```python
from build123d import *

# Parameters (mm, degrees)
F0_W      = 2032
F0_H      = 812.8
F1_DEPTH  = 914.4
F4_DEPTH  = 1955.8
F3_W      = 1879.6
F3_H      = 330.2
F5_DEPTH  = 736.6
F6_W      = 660.4
F6_H      = 241.3
F7_DEPTH  = 736.6
F8_W      = 76.2
F8_H      = 660.4
F10_R     = 76.2
F11_DEPTH = 76.2
F12_DEPTH = 50.8


with BuildPart() as f1:
    # F0 (on Top) → F1 (new body)
    with BuildSketch(Plane.XY):
        Rectangle(F0_W, F0_H)
    extrude(amount=F1_DEPTH)

    # F2 (on face) → F4 (cut)
    with BuildSketch(Plane.YZ.offset(1016)):
        with BuildLine():
            Line((330.2, 63.5), (330.2, 304.8))
            ThreePointArc((330.2, 304.8), (0, 381), (-330.2, 304.8))
            Line((-330.2, 304.8), (-330.2, 63.5))
            Line((-330.2, 63.5), (330.2, 63.5))
        make_face()
    extrude(amount=-F4_DEPTH, mode=Mode.SUBTRACT)

    # F3 (on face) → F5 (cut)
    with BuildSketch(Plane.XZ.offset(406.4)):
        with Locations((0, 698.5)):
            Rectangle(F3_W, F3_H)
    extrude(amount=-F5_DEPTH, mode=Mode.SUBTRACT)

    # F6 (on face) → F7 (cut)
    with BuildSketch(Plane.XZ.offset(406.4)):
        with Locations((-609.6, 184.15)):
            Rectangle(F6_W, F6_H)
        with BuildLine():
            ThreePointArc((-279.4, 304.8), (-609.6, 381), (-939.8, 304.8))
            Line((-939.8, 304.8), (-279.4, 304.8))
        make_face()
    extrude(amount=-F7_DEPTH, mode=Mode.SUBTRACT)

    # F8 (on face) → F9 (join, up to the next surface of F1)
    with BuildSketch(Plane.XY.offset(63.5)):
        with Locations((977.9, 0)):
            Rectangle(F8_W, F8_H)
    extrude(until=Until.NEXT)

    # F10 (on face) → F11 (cut, through all)
    with BuildSketch(Plane.YZ.offset(1016)):
        with Locations((0, 152.4)):
            Circle(F10_R)
    extrude(amount=-F11_DEPTH, mode=Mode.SUBTRACT)

    # F12 (cut): a face of the model
    f12_faces = [f1.faces().sort_by_distance(p)[0] for p in [
        (0, 0, 914.4),
    ]]
    extrude(f12_faces, amount=-F12_DEPTH, mode=Mode.SUBTRACT)


solid = f1.part
```
For this review, take the finished solid that the model builds, in its own axes (mm). A direction names the side the tool comes from. Give positions to 0.01 mm unless a question says otherwise; leave off trailing zeros. Write each loop counter-clockwise with the first axis right and the second up, starting at its lowest first coordinate (ties: lowest second). Pieces come first, ordered by that corner, then holes. Notation, with made-up numbers: M 89.5,43 L 147.5,43 A30 ccw 147.5,76 Z; hole C 26.25,-11.5 d5. An arc over 180 degrees is marked long. Answer as CSV lines item,"result".
1. Consider section C-C, the plane y = -196. Write out the cut boundary in (x, z), then the cut area to 3 significant figures.
Findings:
outline,"M -1016,0 L 1016,0 L 1016,863.6 L 939.8,863.6 L 939.8,533.4 L -939.8,533.4 L -939.8,863.6 L -1016,863.6 Z; hole M -939.8,63.5 L 939.8,63.5 L 939.8,355.06 L -413.6,355.06 A753.53 ccw -805.6,355.06 L -939.8,355.06 Z"
area,"579,000 mm2"
2. Wall thickness on line 1 (X direction, y = -156.5, z = 250); line 2 (Z direction, x = -587, y = 197); line 3 (Y direction, x = -53.5, z = 178.5): over which ranges is each line inside the solid? List them lowest first.
Findings:
line 1,"x = -1016 to -939.8, 939.8 to 1016"
line 2,"z = 0 to 63.5, 380.66 to 533.4"
line 3,"y = -406.4 to -330.2, 330.2 to 406.4"
3. Consider section D-D, the plane z = 683. Write out the cut boundary in (x, y).
Findings:
outline,"M -1016,-406.4 L -939.8,-406.4 L -939.8,330.2 L 939.8,330.2 L 939.8,-406.4 L 1016,-406.4 L 1016,406.4 L -1016,406.4 Z"
4. For faces 4 (the flat face through (-939.8, -43, 220)), 5 (the flat face through (-279.4, -369, 182)), 6 (the flat face through (-13, -43, 533.4)), list the 3-axis set-ups (+Z, -Z, +X, -X, +Y, -Y) from which the entire face can be reached by the end or side of a thin tool; tool diameter is ignored.
Findings:
face 4,"none"
face 5,"-Y"
face 6,"+Z, -Y"
5. Consider section B-B, the plane z = 203.5. Write out the cut boundary in (x, y).
Findings:
outline,"M -1016,-406.4 L -939.8,-406.4 L -939.8,330.2 L 939.8,330.2 L 939.8,56.53 L 1016,56.53 L 1016,406.4 L -1016,406.4 Z; M -279.4,-406.4 L 1016,-406.4 L 1016,-56.53 L 939.8,-56.53 L 939.8,-330.2 L -279.4,-330.2 Z"
6. Draft analysis for pull direction Y (two halves, no side actions). For faces 1 (the flat face through (-14, -406.4, 330)), 2 (the flat face through (939.8, -43, 696)), 3 (the flat face through (-13, -43, 63.5)), state which applies: +Y half, -Y half, draft (parallel to the pull), parting line (faces both ways), or undercut.
Findings:
face 1,"-Y half"
face 2,"draft"
face 3,"undercut"
7. Consider section A-A, the plane x = 426. Write out the cut boundary in (y, z), then the cut area to 3 significant figures.
Findings:
outline,"M -406.4,0 L 406.4,0 L 406.4,863.6 L 330.2,863.6 L 330.2,533.4 L -406.4,533.4 Z; hole M -330.2,63.5 L 330.2,63.5 L 330.2,304.8 A753.53 ccw -330.2,304.8 Z"
area,"265,000 mm2"
8. For pin 1 (8 mm diameter, centred on x = -240, z = 760, fed in from -Y); pin 2 (1.5 mm diameter, centred on x = 228.5, y = 291.5, fed in from +Z), all flat-tipped, find the tip position at first contact; note any pin that passes through.
Findings:
pin 1,"stops at y = 330.2"
pin 2,"stops at z = 533.4"
